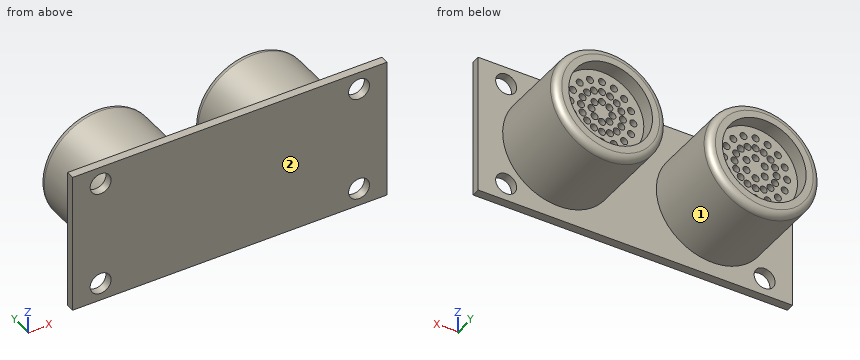
from build123d import *

# Parameters (mm, degrees)
SKETCH_1_W          = 45
SKETCH_1_H          = 20
EXTRUDE_1_DEPTH     = 1.2
SKETCH_2_R          = 8
SKETCH_2_R_2        = 6
EXTRUDE_2_DEPTH     = 12
FILLET_1_R          = 1
EXTRUDE_START       = -8
SKETCH_3_R          = 6
SKETCH_3_R_2        = 0.5
EXTRUDE_3_DEPTH     = 8
SKETCH_4_R          = 0.5
CUT_EXTRUDE_1_DEPTH = 8
SKETCH_5_R          = 1.5
CUT_EXTRUDE_2_DEPTH = 28.39069185


with BuildPart() as part:
    # 草图1 → 凸台-拉伸1 (new body)
    with BuildSketch(Plane(origin=(0, 0, 0), x_dir=(1, 0, 0), z_dir=(0, 1, 0))):
        Rectangle(SKETCH_1_W, SKETCH_1_H)
    extrude(amount=EXTRUDE_1_DEPTH)

    # 草图2 → 凸台-拉伸2 (add)
    # profile 1 of 2: a face of its own
    with BuildSketch(Plane(origin=(0, 1.2, 0), x_dir=(1, 0, 0), z_dir=(0, 1, 0))):
        with Locations(Location((-11, 0, 0), (0, 0, 270))):
            Circle(SKETCH_2_R)
        with Locations(Location((-11, 0, 0), (0, 0, 270))):
            Circle(SKETCH_2_R_2, mode=Mode.SUBTRACT)
    # profile 2 of 2: a face of its own
    with BuildSketch(Plane(origin=(0, 1.2, 0), x_dir=(1, 0, 0), z_dir=(0, 1, 0))):
        with Locations(Location((11, 0, 0), (0, 0, 270))):
            Circle(SKETCH_2_R)
        with Locations(Location((11, 0, 0), (0, 0, 270))):
            Circle(SKETCH_2_R_2, mode=Mode.SUBTRACT)
    extrude(amount=EXTRUDE_2_DEPTH)

    # 圆角1
    fillet_1_edges = [part.edges().sort_by_distance(p)[0] for p in [
        (-11, 13.2, -8),
        (11, 13.2, -8),
    ]]
    fillet(fillet_1_edges, radius=FILLET_1_R)

    # 草图3 → 凸台-拉伸3 (add)
    # profile 1 of 2: a face of its own
    with BuildSketch(Plane(origin=(0, 11.2, 0), x_dir=(1, 0, 0), z_dir=(0, 1, 0)).offset(EXTRUDE_START)):
        with Locations(Location((-11, 0, 0), (0, 0, 270))):
            Circle(SKETCH_3_R)
        with Locations(Location((-11, 4.509880422, 0), (0, 0, 270))):
            Circle(SKETCH_3_R_2, mode=Mode.SUBTRACT)
        with Locations(Location((-11, 3.009880422, 0), (0, 0, 270))):
            Circle(SKETCH_3_R_2, mode=Mode.SUBTRACT)
        with Locations(Location((-11, 1.509880422, 0), (0, 0, 270))):
            Circle(SKETCH_3_R_2, mode=Mode.SUBTRACT)
        with Locations(Location((-9.27414348, 4.166586216, 0), (0, 0, 270))):
            Circle(SKETCH_3_R_2, mode=Mode.SUBTRACT)
        with Locations(Location((-9.848168629, 2.780766918, 0), (0, 0, 270))):
            Circle(SKETCH_3_R_2, mode=Mode.SUBTRACT)
        with Locations(Location((-7.811032971, 3.188967029, 0), (0, 0, 270))):
            Circle(SKETCH_3_R_2, mode=Mode.SUBTRACT)
        with Locations(Location((-8.871693143, 2.128306857, 0), (0, 0, 270))):
            Circle(SKETCH_3_R_2, mode=Mode.SUBTRACT)
        with Locations(Location((-6.833413784, 1.72585652, 0), (0, 0, 270))):
            Circle(SKETCH_3_R_2, mode=Mode.SUBTRACT)
        with Locations(Location((-8.219233082, 1.151831371, 0), (0, 0, 270))):
            Circle(SKETCH_3_R_2, mode=Mode.SUBTRACT)
        with Locations(Location((-6.490119578, 0, 0), (0, 0, 270))):
            Circle(SKETCH_3_R_2, mode=Mode.SUBTRACT)
        with Locations(Location((-7.990119578, 0, 0), (0, 0, 270))):
            Circle(SKETCH_3_R_2, mode=Mode.SUBTRACT)
        with Locations(Location((-6.833413784, -1.72585652, 0), (0, 0, 270))):
            Circle(SKETCH_3_R_2, mode=Mode.SUBTRACT)
        with Locations(Location((-8.219233082, -1.151831371, 0), (0, 0, 270))):
            Circle(SKETCH_3_R_2, mode=Mode.SUBTRACT)
        with Locations(Location((-7.811032971, -3.188967029, 0), (0, 0, 270))):
            Circle(SKETCH_3_R_2, mode=Mode.SUBTRACT)
        with Locations(Location((-8.871693143, -2.128306857, 0), (0, 0, 270))):
            Circle(SKETCH_3_R_2, mode=Mode.SUBTRACT)
        with Locations(Location((-9.27414348, -4.166586216, 0), (0, 0, 270))):
            Circle(SKETCH_3_R_2, mode=Mode.SUBTRACT)
        with Locations(Location((-9.848168629, -2.780766918, 0), (0, 0, 270))):
            Circle(SKETCH_3_R_2, mode=Mode.SUBTRACT)
        with Locations(Location((-11, -4.509880422, 0), (0, 0, 270))):
            Circle(SKETCH_3_R_2, mode=Mode.SUBTRACT)
        with Locations(Location((-11, -3.009880422, 0), (0, 0, 270))):
            Circle(SKETCH_3_R_2, mode=Mode.SUBTRACT)
        with Locations(Location((-12.72585652, -4.166586216, 0), (0, 0, 270))):
            Circle(SKETCH_3_R_2, mode=Mode.SUBTRACT)
        with Locations(Location((-12.151831371, -2.780766918, 0), (0, 0, 270))):
            Circle(SKETCH_3_R_2, mode=Mode.SUBTRACT)
        with Locations(Location((-14.188967029, -3.188967029, 0), (0, 0, 270))):
            Circle(SKETCH_3_R_2, mode=Mode.SUBTRACT)
        with Locations(Location((-13.128306857, -2.128306857, 0), (0, 0, 270))):
            Circle(SKETCH_3_R_2, mode=Mode.SUBTRACT)
        with Locations(Location((-15.166586216, -1.72585652, 0), (0, 0, 270))):
            Circle(SKETCH_3_R_2, mode=Mode.SUBTRACT)
        with Locations(Location((-13.780766918, -1.151831371, 0), (0, 0, 270))):
            Circle(SKETCH_3_R_2, mode=Mode.SUBTRACT)
        with Locations(Location((-15.509880422, 0, 0), (0, 0, 270))):
            Circle(SKETCH_3_R_2, mode=Mode.SUBTRACT)
        with Locations(Location((-14.009880422, 0, 0), (0, 0, 270))):
            Circle(SKETCH_3_R_2, mode=Mode.SUBTRACT)
        with Locations(Location((-15.166586216, 1.72585652, 0), (0, 0, 270))):
            Circle(SKETCH_3_R_2, mode=Mode.SUBTRACT)
        with Locations(Location((-13.780766918, 1.151831371, 0), (0, 0, 270))):
            Circle(SKETCH_3_R_2, mode=Mode.SUBTRACT)
        with Locations(Location((-14.188967029, 3.188967029, 0), (0, 0, 270))):
            Circle(SKETCH_3_R_2, mode=Mode.SUBTRACT)
        with Locations(Location((-13.128306857, 2.128306857, 0), (0, 0, 270))):
            Circle(SKETCH_3_R_2, mode=Mode.SUBTRACT)
        with Locations(Location((-12.72585652, 4.166586216, 0), (0, 0, 270))):
            Circle(SKETCH_3_R_2, mode=Mode.SUBTRACT)
        with Locations(Location((-12.151831371, 2.780766918, 0), (0, 0, 270))):
            Circle(SKETCH_3_R_2, mode=Mode.SUBTRACT)
        with Locations(Location((-9.692405197, 0.754940211, 0), (0, 0, 270))):
            Circle(SKETCH_3_R_2, mode=Mode.SUBTRACT)
        with Locations(Location((-9.692405197, -0.754940211, 0), (0, 0, 270))):
            Circle(SKETCH_3_R_2, mode=Mode.SUBTRACT)
        with Locations(Location((-11, -1.509880422, 0), (0, 0, 270))):
            Circle(SKETCH_3_R_2, mode=Mode.SUBTRACT)
        with Locations(Location((-12.307594803, -0.754940211, 0), (0, 0, 270))):
            Circle(SKETCH_3_R_2, mode=Mode.SUBTRACT)
        with Locations(Location((-12.307594803, 0.754940211, 0), (0, 0, 270))):
            Circle(SKETCH_3_R_2, mode=Mode.SUBTRACT)
    # profile 2 of 2: a face of its own
    with BuildSketch(Plane(origin=(0, 11.2, 0), x_dir=(1, 0, 0), z_dir=(0, 1, 0)).offset(EXTRUDE_START)):
        with Locations(Location((11, 0, 0), (0, 0, 270))):
            Circle(SKETCH_3_R)
    extrude(amount=EXTRUDE_3_DEPTH)

    # 草图4 → 切除-拉伸1 (cut)
    with BuildSketch(Plane(origin=(0, 11.2, 0), x_dir=(1, 0, 0), z_dir=(0, 1, 0))):
        with Locations(Location((11, 1.5, 0), (0, 0, 270))):
            Circle(SKETCH_4_R)
        with Locations(Location((11, 3, 0), (0, 0, 270))):
            Circle(SKETCH_4_R)
        with Locations(Location((11, 4.5, 0), (0, 0, 270))):
            Circle(SKETCH_4_R)
        with Locations(Location((12.722075446, 4.157457896, 0), (0, 0, 270))):
            Circle(SKETCH_4_R)
        with Locations(Location((12.148050297, 2.771638598, 0), (0, 0, 270))):
            Circle(SKETCH_4_R)
        with Locations(Location((14.181980515, 3.181980515, 0), (0, 0, 270))):
            Circle(SKETCH_4_R)
        with Locations(Location((13.121320344, 2.121320344, 0), (0, 0, 270))):
            Circle(SKETCH_4_R)
        with Locations(Location((15.157457896, 1.722075446, 0), (0, 0, 270))):
            Circle(SKETCH_4_R)
        with Locations(Location((13.771638598, 1.148050297, 0), (0, 0, 270))):
            Circle(SKETCH_4_R)
        with Locations(Location((15.5, 0, 0), (0, 0, 270))):
            Circle(SKETCH_4_R)
        with Locations(Location((14, 0, 0), (0, 0, 270))):
            Circle(SKETCH_4_R)
        with Locations(Location((15.157457896, -1.722075446, 0), (0, 0, 270))):
            Circle(SKETCH_4_R)
        with Locations(Location((13.771638598, -1.148050297, 0), (0, 0, 270))):
            Circle(SKETCH_4_R)
        with Locations(Location((14.181980515, -3.181980515, 0), (0, 0, 270))):
            Circle(SKETCH_4_R)
        with Locations(Location((13.121320344, -2.121320344, 0), (0, 0, 270))):
            Circle(SKETCH_4_R)
        with Locations(Location((12.722075446, -4.157457896, 0), (0, 0, 270))):
            Circle(SKETCH_4_R)
        with Locations(Location((12.148050297, -2.771638598, 0), (0, 0, 270))):
            Circle(SKETCH_4_R)
        with Locations(Location((11, -4.5, 0), (0, 0, 270))):
            Circle(SKETCH_4_R)
        with Locations(Location((11, -3, 0), (0, 0, 270))):
            Circle(SKETCH_4_R)
        with Locations(Location((9.277924554, -4.157457896, 0), (0, 0, 270))):
            Circle(SKETCH_4_R)
        with Locations(Location((9.851949703, -2.771638598, 0), (0, 0, 270))):
            Circle(SKETCH_4_R)
        with Locations(Location((7.818019485, -3.181980515, 0), (0, 0, 270))):
            Circle(SKETCH_4_R)
        with Locations(Location((8.878679656, -2.121320344, 0), (0, 0, 270))):
            Circle(SKETCH_4_R)
        with Locations(Location((6.842542104, -1.722075446, 0), (0, 0, 270))):
            Circle(SKETCH_4_R)
        with Locations(Location((8.228361402, -1.148050297, 0), (0, 0, 270))):
            Circle(SKETCH_4_R)
        with Locations(Location((6.5, 0, 0), (0, 0, 270))):
            Circle(SKETCH_4_R)
        with Locations(Location((8, 0, 0), (0, 0, 270))):
            Circle(SKETCH_4_R)
        with Locations(Location((6.842542104, 1.722075446, 0), (0, 0, 270))):
            Circle(SKETCH_4_R)
        with Locations(Location((8.228361402, 1.148050297, 0), (0, 0, 270))):
            Circle(SKETCH_4_R)
        with Locations(Location((7.818019485, 3.181980515, 0), (0, 0, 270))):
            Circle(SKETCH_4_R)
        with Locations(Location((8.878679656, 2.121320344, 0), (0, 0, 270))):
            Circle(SKETCH_4_R)
        with Locations(Location((9.277924554, 4.157457896, 0), (0, 0, 270))):
            Circle(SKETCH_4_R)
        with Locations(Location((9.851949703, 2.771638598, 0), (0, 0, 270))):
            Circle(SKETCH_4_R)
        with Locations(Location((12.060660172, 1.060660172, 0), (0, 0, 270))):
            Circle(SKETCH_4_R)
        with Locations(Location((12.5, 0, 0), (0, 0, 270))):
            Circle(SKETCH_4_R)
        with Locations(Location((12.060660172, -1.060660172, 0), (0, 0, 270))):
            Circle(SKETCH_4_R)
        with Locations(Location((11, -1.5, 0), (0, 0, 270))):
            Circle(SKETCH_4_R)
        with Locations(Location((9.939339828, -1.060660172, 0), (0, 0, 270))):
            Circle(SKETCH_4_R)
        with Locations(Location((9.5, 0, 0), (0, 0, 270))):
            Circle(SKETCH_4_R)
        with Locations(Location((9.939339828, 1.060660172, 0), (0, 0, 270))):
            Circle(SKETCH_4_R)
    extrude(amount=-CUT_EXTRUDE_1_DEPTH, mode=Mode.SUBTRACT)

    # 草图5 → 切除-拉伸2 (cut, through all)
    with BuildSketch(Plane(origin=(0, 1.2, 0), x_dir=(1, 0, 0), z_dir=(0, 1, 0))):
        with Locations(Location((-18.5, 7.5, 0), (0, 0, 270))):
            Circle(SKETCH_5_R)
        with Locations(Location((-18.5, -7.5, 0), (0, 0, 90))):
            Circle(SKETCH_5_R)
        with Locations(Location((18.5, -7.5, 0), (0, 0, 270))):
            Circle(SKETCH_5_R)
        with Locations(Location((18.5, 7.5, 0), (0, 0, 90))):
            Circle(SKETCH_5_R)
    extrude(amount=-CUT_EXTRUDE_2_DEPTH, mode=Mode.SUBTRACT)


solid = part.part
For this review, take the finished solid that the model builds, in its own axes (mm). Face numbers are marked on the shaded views. Give positions to 0.01 mm unless a question says otherwise; leave off trailing zeros. Answer as a JSON object with one key per item and string values. Group by question number.
Item 1: Take a section at A-A on x = 11. Give the number of separate pieces and of enclosed holes in the cut face, and give its area (3 significant figures).
Item 2: Clearance check with flat-ended pins moving along their axes: pin 1 Ø8 at (x, z) = (11.5, -1.5) entering from -Y; pin 2 Ø3.5 at (x, z) = (-9, 2.5) entering from +Y; pin 3 Ø6 at (x, y) = (17, 6) entering from +Z; pin 4 Ø2 at (y, z) = (11, -4) entering from -X. State where each tip first meets the part, or that it passes through.
Item 3: Wall thickness on line 1 along X through (y, z) = (11.5, 1.75); line 2 along X through (y, z) = (2, 1); line 3 along Y through (x, z) = (-13.5, 3.25): over which ranges is each line inside the solid? List them lowest first.
Item 4: Draft analysis for pull direction X (two halves, no side actions). For the marked faces 1 and 2, state which applies: pulls with the +X half, pulls with the -X half, needs draft (parallel to the pull), parting line crosses it, or undercut.
Reported:
{
 "1": {"separate pieces": "6", "enclosed holes": "0", "area": "120 mm^2"},
 "2": {"pin 1": "y = 0", "pin 2": "y = 11.2", "pin 3": "z = 7.42", "pin 4": "x = -18.42"},
 "3": {"line 1": "-18.81 to -16.74, -5.26 to -3.19, 3.19 to 5.26, 16.74 to 18.81", "line 2": "-18.94 to -16.92, -5.08 to -3.06, 3.06 to 5.08, 16.92 to 18.94", "line 3": "0 to 1.2, 3.2 to 11.2"},
 "4": {"face 1": "undercut", "face 2": "needs draft"}
}
